Read the model definition and answer for the solid it produces. Units are mm, in the model's axes. Face numbers are marked on the shaded views. A direction names the side the tool comes from. Round coordinates to 2 decimals unless told otherwise and drop trailing zeros. Loops run counter-clockwise (first coordinate to the right, second up) from the corner with the lowest first, then second, coordinate; pieces in that order, holes last. Notation, with made-up numbers: M 56,-5 L 94,-5 A19 cw 94,10 Z; hole C -17.5,-39 d3. An arc over 180 degrees is marked long. Write each question's results on one line, items separated by ' | '.
from build123d import *
from OCP.BRepFilletAPI import BRepFilletAPI_MakeChamfer

# Parameters (mm, degrees)
PIPESKETCH_R        = 5.1435
PIPESKETCH_R_2      = 1.0795
EXTRUSION_DEPTH     = 34.036
SKETCH1_R           = 1.0795
BOSS_EXTRUDE1_DEPTH = 5.08
SKETCH9_R           = 3.4163
CUT_EXTRUDE1_DEPTH  = 9.906
CHAMFER1_SIZE       = 0.254
CHAMFER1_SIZE2      = 0.262273252


with BuildPart() as part:
    # PipeSketch → Extrusion (new body)
    with BuildSketch(Plane.XY):
        Circle(PIPESKETCH_R)
        Circle(PIPESKETCH_R_2, mode=Mode.SUBTRACT)
    extrude(amount=EXTRUSION_DEPTH)

    # Sketch1 → Boss-Extrude1 (add)
    with BuildSketch(Plane.XY.offset(19.05)):
        Polygon((5.1435, 2.96960111), (0, 5.939202219), (-5.1435, 2.96960111), (-5.1435, -2.96960111), (0, -5.939202219), (5.1435, -2.96960111), align=None)
        Circle(SKETCH1_R, mode=Mode.SUBTRACT)
    extrude(amount=BOSS_EXTRUDE1_DEPTH)

    # Sketch9 → Cut-Extrude1 (cut)
    with BuildSketch(Plane.XY.offset(34.036)):
        Circle(SKETCH9_R)
    extrude(amount=-CUT_EXTRUDE1_DEPTH, mode=Mode.SUBTRACT)

    # Sketch7 → Cut-Revolve7 (revolve, cut)
    with BuildSketch(Plane(origin=(0, 0, 0), x_dir=(0, 0, -1), z_dir=(1, 0, 0)), mode=Mode.PRIVATE) as cut_revolve7_sk:
        Polygon((-34.036, 5.1435), (-34.036, 4.839599393), (-24.257, 5.1435), align=None)
        Polygon((0, 5.1435), (-19.05, 5.1435), (-19.05, 1.5875), (-18.923, 1.5875), (-14.19225, 1.3335), (-14.19225, 1.5875), (-9.4615, 1.3335), (-9.4615, 1.5875), (-4.73075, 1.3335), (-4.73075, 1.5875), (0, 1.3335), align=None)
    revolve(cut_revolve7_sk.sketch.rotate(Axis((0, 0, 0), (0, 0, -1)), 90), axis=Axis((0, 0, 0), (0, 0, -1)), mode=Mode.SUBTRACT)

    # Sketch4 → Cut-Revolve6 (revolve, cut)
    with BuildSketch(Plane(origin=(0, 0, 0), x_dir=(1, 0, 0), z_dir=(0, 1, 0))):
        Polygon((-5.1435, -24.13), (-14.0335, -24.13), (-14.0335, -22.225), align=None)
        Polygon((-5.1435, -19.05), (-14.0335, -19.05), (-14.0335, -20.955), align=None)
    revolve(axis=Axis((0, 0, 0), (0, 0, 1)), mode=Mode.SUBTRACT)

    # Chamfer1: one chamfer whose edges measure the first distance from different faces: ONE call of the kernel's chamfer builder (chamfer() names one face for all edges)
    chamfer1_edges_1 = [part.edges().sort_by_distance(p)[0] for p in [
        (-3.4163, 0, 34.036),
    ]]
    chamfer1_edges_2 = [part.edges().sort_by_distance(p)[0] for p in [
        (-4.839599393, 0, 34.036),
    ]]
    chamfer1_side_2 = [part.faces().sort_by_distance(p)[0] for p in [
        (-4.991549697, 0, 29.1465),
    ]]
    chamfer1 = BRepFilletAPI_MakeChamfer(part.part.solid().wrapped)
    for e in chamfer1_edges_1:
        chamfer1.Add(CHAMFER1_SIZE, e.wrapped)
    for e in chamfer1_edges_2:
        chamfer1.Add(CHAMFER1_SIZE, CHAMFER1_SIZE2, e.wrapped, chamfer1_side_2[0].wrapped)  # the first distance lies on this face
    add(Compound.cast(chamfer1.Shape()), mode=Mode.REPLACE)


solid = part.part
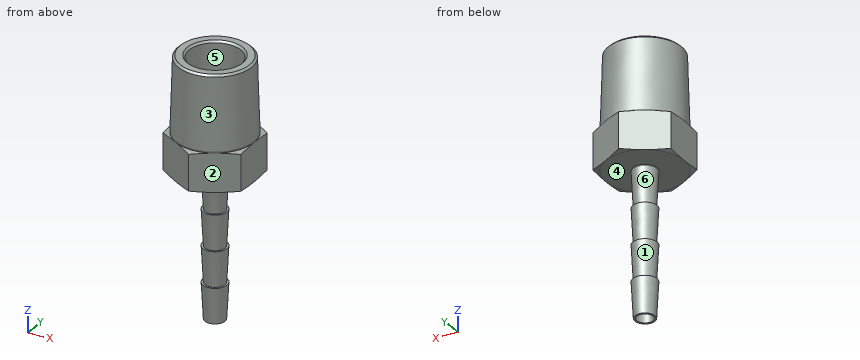
Item 1: The mould has two halves that part along X. Classify the marked faces 4, 5 and 6: pulls with the +X half, pulls with the -X half, needs draft (parallel to the pull), parting line crosses it, or undercut.
Outcome:
face 4: needs draft | face 5: undercut | face 6: parting line crosses it
Item 2: For the marked faces 1, 2 and 3, determine the directions among +Z, -Z, +X, -X, +Y, -Y from which every point of the face is accessible in a straight line to the end or side of a thin tool.
Outcome:
face 1: none | face 2: +Z, -Z, +X, -Y | face 3: +Z
Item 3: The part is cut by section C-C (z = 14.5). Determine the outline of the cut face in (x, y), plus the area to 3 significant figures.
Outcome:
outline: C 0,0 d2.7; hole C 0,0 d2.16 | area: 2.06 mm2
Item 4: The part is cut by section A-A (z = 22.5). Determine the outline of the cut face in (x, y).
Outcome:
outline: M -5.14,-2.97 L 0,-5.94 L 5.14,-2.97 L 5.14,2.97 L 0,5.94 L -5.14,2.97 Z; hole C 0,0 d2.16
Item 5: Flat-ended cylindrical pins translate along their axes: pin 1 (6 mm diameter, centred on y = -4, z = 23, fed in from -X); pin 2 (1 mm diameter, centred on x = 4, z = 18, fed in from -Y); pin 3 (2.5 mm diameter, centred on x = -1, y = -0.5, fed in from +Z); pin 4 (3 mm diameter, centred on x = -3, y = 1, fed in from -Z). Find the tip coordinate at first contact, or state that the pin passes through.
Outcome:
pin 1: stops at x = -5.14 | pin 2: passes through | pin 3: stops at z = 24.13 | pin 4: stops at z = 19.05
Item 6: The part is cut by section B-B (z = 3). Determine the outline of the cut face in (x, y), plus the area to 3 significant figures.
Outcome:
outline: C 0,0 d2.99; hole C 0,0 d2.16 | area: 3.36 mm2
Item 7: Straight lines are drawn through the part: line 1 (Z direction, x = -2, y = -1.5); line 2 (Z direction, x = 2.5, y = -3); line 3 (Y direction, x = 0, z = 9.75). For each, find the intervals that lie inside material, in ascending order.
Outcome:
line 1: z = 19.05 to 24.13 | line 2: z = 19.05 to 34.04 | line 3: y = -1.35 to -1.08, 1.08 to 1.35
